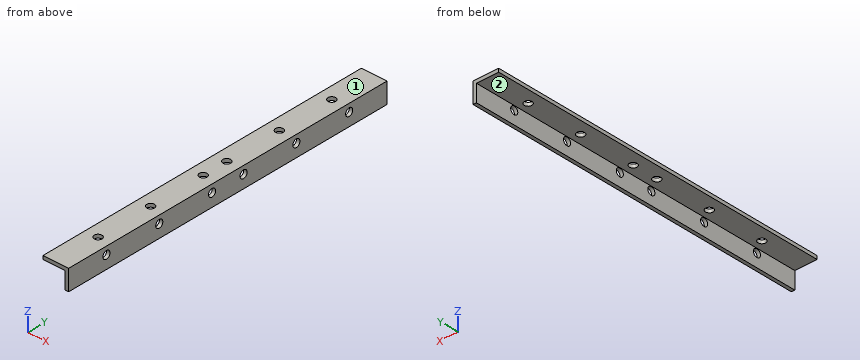
from build123d import *

# Parameters (mm, degrees)
BOSS_EXTRUDE1_DEPTH = 202
CUT_EXTRUDE1_REACH  = 14
SKETCH2_R           = 2.25
CUT_EXTRUDE2_REACH  = 17
SKETCH3_R           = 2.25


with BuildPart() as part:
    # Sketch1 → Boss-Extrude1 (new body)
    with BuildSketch(Plane(origin=(0, 0, 0), x_dir=(1, 0, 0), z_dir=(0, 1, 0))):
        Polygon((0, 0), (15, 0), (15, 12), (13, 12), (13, 2), (0, 2), align=None)
    extrude(amount=BOSS_EXTRUDE1_DEPTH)

    # Sketch2 → Cut-Extrude1 (cut, up to next)
    with BuildSketch(Plane.XY, mode=Mode.PRIVATE) as cut_extrude1_sk1:
        with Locations((7.5, 175.166666667)):
            Circle(SKETCH2_R)
    cut_extrude1_tool1 = extrude(cut_extrude1_sk1.sketch, amount=-CUT_EXTRUDE1_REACH, mode=Mode.PRIVATE) & part.part
    add(cut_extrude1_tool1.solids().sort_by_distance((7.5, 175.166667, 0))[0], mode=Mode.SUBTRACT)
    # Sketch2 → Cut-Extrude1 (cut, up to next)
    with BuildSketch(Plane.XY, mode=Mode.PRIVATE) as cut_extrude1_sk2:
        with Locations((7.5, 141.833333333)):
            Circle(SKETCH2_R)
    cut_extrude1_tool2 = extrude(cut_extrude1_sk2.sketch, amount=-CUT_EXTRUDE1_REACH, mode=Mode.PRIVATE) & part.part
    add(cut_extrude1_tool2.solids().sort_by_distance((7.5, 141.833333, 0))[0], mode=Mode.SUBTRACT)
    # Sketch2 → Cut-Extrude1 (cut, up to next)
    with BuildSketch(Plane.XY, mode=Mode.PRIVATE) as cut_extrude1_sk3:
        with Locations((7.5, 108.5)):
            Circle(SKETCH2_R)
    cut_extrude1_tool3 = extrude(cut_extrude1_sk3.sketch, amount=-CUT_EXTRUDE1_REACH, mode=Mode.PRIVATE) & part.part
    add(cut_extrude1_tool3.solids().sort_by_distance((7.5, 108.5, 0))[0], mode=Mode.SUBTRACT)
    # Sketch2 → Cut-Extrude1 (cut, up to next)
    with BuildSketch(Plane.XY, mode=Mode.PRIVATE) as cut_extrude1_sk4:
        with Locations((7.5, 93.5)):
            Circle(SKETCH2_R)
    cut_extrude1_tool4 = extrude(cut_extrude1_sk4.sketch, amount=-CUT_EXTRUDE1_REACH, mode=Mode.PRIVATE) & part.part
    add(cut_extrude1_tool4.solids().sort_by_distance((7.5, 93.5, 0))[0], mode=Mode.SUBTRACT)
    # Sketch2 → Cut-Extrude1 (cut, up to next)
    with BuildSketch(Plane.XY, mode=Mode.PRIVATE) as cut_extrude1_sk5:
        with Locations((7.5, 60.166666667)):
            Circle(SKETCH2_R)
    cut_extrude1_tool5 = extrude(cut_extrude1_sk5.sketch, amount=-CUT_EXTRUDE1_REACH, mode=Mode.PRIVATE) & part.part
    add(cut_extrude1_tool5.solids().sort_by_distance((7.5, 60.166667, 0))[0], mode=Mode.SUBTRACT)
    # Sketch2 → Cut-Extrude1 (cut, up to next)
    with BuildSketch(Plane.XY, mode=Mode.PRIVATE) as cut_extrude1_sk6:
        with Locations((7.5, 26.833333333)):
            Circle(SKETCH2_R)
    cut_extrude1_tool6 = extrude(cut_extrude1_sk6.sketch, amount=-CUT_EXTRUDE1_REACH, mode=Mode.PRIVATE) & part.part
    add(cut_extrude1_tool6.solids().sort_by_distance((7.5, 26.833333, 0))[0], mode=Mode.SUBTRACT)

    # Sketch3 → Cut-Extrude2 (cut, up to next)
    with BuildSketch(Plane(origin=(15, 0, 0), x_dir=(0, 0, -1), z_dir=(1, 0, 0)), mode=Mode.PRIVATE) as cut_extrude2_sk1:
        with Locations((4.5, 24)):
            Circle(SKETCH3_R)
    cut_extrude2_tool1 = extrude(cut_extrude2_sk1.sketch, amount=-CUT_EXTRUDE2_REACH, mode=Mode.PRIVATE) & part.part
    add(cut_extrude2_tool1.solids().sort_by_distance((15, 24, -4.5))[0], mode=Mode.SUBTRACT)
    # Sketch3 → Cut-Extrude2 (cut, up to next)
    with BuildSketch(Plane(origin=(15, 0, 0), x_dir=(0, 0, -1), z_dir=(1, 0, 0)), mode=Mode.PRIVATE) as cut_extrude2_sk2:
        with Locations((4.5, 57.5)):
            Circle(SKETCH3_R)
    cut_extrude2_tool2 = extrude(cut_extrude2_sk2.sketch, amount=-CUT_EXTRUDE2_REACH, mode=Mode.PRIVATE) & part.part
    add(cut_extrude2_tool2.solids().sort_by_distance((15, 57.5, -4.5))[0], mode=Mode.SUBTRACT)
    # Sketch3 → Cut-Extrude2 (cut, up to next)
    with BuildSketch(Plane(origin=(15, 0, 0), x_dir=(0, 0, -1), z_dir=(1, 0, 0)), mode=Mode.PRIVATE) as cut_extrude2_sk3:
        with Locations((4.5, 91)):
            Circle(SKETCH3_R)
    cut_extrude2_tool3 = extrude(cut_extrude2_sk3.sketch, amount=-CUT_EXTRUDE2_REACH, mode=Mode.PRIVATE) & part.part
    add(cut_extrude2_tool3.solids().sort_by_distance((15, 91, -4.5))[0], mode=Mode.SUBTRACT)
    # Sketch3 → Cut-Extrude2 (cut, up to next)
    with BuildSketch(Plane(origin=(15, 0, 0), x_dir=(0, 0, -1), z_dir=(1, 0, 0)), mode=Mode.PRIVATE) as cut_extrude2_sk4:
        with Locations((4.5, 111)):
            Circle(SKETCH3_R)
    cut_extrude2_tool4 = extrude(cut_extrude2_sk4.sketch, amount=-CUT_EXTRUDE2_REACH, mode=Mode.PRIVATE) & part.part
    add(cut_extrude2_tool4.solids().sort_by_distance((15, 111, -4.5))[0], mode=Mode.SUBTRACT)
    # Sketch3 → Cut-Extrude2 (cut, up to next)
    with BuildSketch(Plane(origin=(15, 0, 0), x_dir=(0, 0, -1), z_dir=(1, 0, 0)), mode=Mode.PRIVATE) as cut_extrude2_sk5:
        with Locations((4.5, 144.5)):
            Circle(SKETCH3_R)
    cut_extrude2_tool5 = extrude(cut_extrude2_sk5.sketch, amount=-CUT_EXTRUDE2_REACH, mode=Mode.PRIVATE) & part.part
    add(cut_extrude2_tool5.solids().sort_by_distance((15, 144.5, -4.5))[0], mode=Mode.SUBTRACT)
    # Sketch3 → Cut-Extrude2 (cut, up to next)
    with BuildSketch(Plane(origin=(15, 0, 0), x_dir=(0, 0, -1), z_dir=(1, 0, 0)), mode=Mode.PRIVATE) as cut_extrude2_sk6:
        with Locations((4.5, 178)):
            Circle(SKETCH3_R)
    cut_extrude2_tool6 = extrude(cut_extrude2_sk6.sketch, amount=-CUT_EXTRUDE2_REACH, mode=Mode.PRIVATE) & part.part
    add(cut_extrude2_tool6.solids().sort_by_distance((15, 178, -4.5))[0], mode=Mode.SUBTRACT)


solid = part.part
Geometry check sheet. Reference: the model listing, model coordinates, mm. Face numbers are marked on the shaded views. A direction names the side the tool comes from. Give positions to 0.01 mm unless a question says otherwise; leave off trailing zeros. Loops run counter-clockwise (first coordinate to the right, second up) from the corner with the lowest first, then second, coordinate; pieces in that order, holes last. Notation, with made-up numbers: M 5,20 L 24,20 A9 ccw 24,32 Z; hole C 80.25,-7 d1. An arc over 180 degrees is marked long. Answer as a JSON object with one key per item and string values. Group by question number.
Item 1: Sectioned sample at C-C on z = -10.25. Record the boundary of the cut face in (x, y), plus the area to 3 significant figures.
Item 2: Sectioned sample at B-B on y = 85. Record the boundary of the cut face in (x, z).
Item 3: Gauge pin test, flat ends, axial feed: pin 1 (4 mm diameter, centred on y = 178, z = -4.5, fed in from -X); pin 2 (6 mm diameter, centred on x = 7.5, y = 141.83, fed in from -Z); pin 3 (5 mm diameter, centred on y = 106, z = -9.5, fed in from -X). Record the tip position at first contact, or that the pin passes through.
Item 4: Material ranges on L1, parallel to Z at x = 6, y = 193; L2, parallel to X at y = 76, z = -8.5, recorded low to high.
Item 5: Sectioned sample at A-A on x = 3.25. Record the boundary of the cut face in (y, z).
Item 6: Access from +Z, -Z, +X, -X, +Y, -Y to the whole of each face (thin tool, end or side, straight path). Record for the marked faces 1 and 2.
Findings below:
{
 "1": {"outline": "M 13,0 L 15,0 L 15,202 L 13,202 Z", "area": "404 mm2"},
 "2": {"outline": "M 0,-2 L 13,-2 L 13,-12 L 15,-12 L 15,0 L 0,0 Z"},
 "3": {"pin 1": "through", "pin 2": "z = -2", "pin 3": "x = 13"},
 "4": {"L1": "-2 to 0", "L2": "13 to 15"},
 "5": {"outline": "M 0,-2 L 202,-2 L 202,0 L 0,0 Z"},
 "6": {"face 1": "+Z, +X, -X, +Y, -Y", "face 2": "-Z, -X, +Y, -Y"}
}
